Build history of the part. All positions in model axes, mm. Face numbers are marked on the shaded views. Round coordinates to 2 decimals unless told otherwise and drop trailing zeros. Order: outer loops, then holes, each group sorted by start corner. A loop starts at its lowest first (then second) coordinate and runs counter-clockwise, first axis right, second up. Notation, with made-up numbers: M -21.5,56 L -2.5,56 A24 ccw -2.5,88 Z; hole C -30.75,88 d3. An arc over 180 degrees is marked long. Use CSV: the item, a comma, the result in double quotes.
from build123d import *

# Parameters (mm, degrees)
PAD_DEPTH   = 40
SKETCH001_R = 5.5
HOLE_DEPTH  = 40.001


with BuildPart() as part:
    # Sketch → Pad (new body)
    with BuildSketch(Plane.XY):
        with BuildLine():
            Line((-17.5, 0), (-17.5, -17.5))
            Line((-17.5, -17.5), (17.5, -17.5))
            Line((17.5, -17.5), (17.5, 0))
            ThreePointArc((17.5, 0), (0, 17.5), (-17.5, 0))
        make_face()
    extrude(amount=PAD_DEPTH)

    # Sketch001 (on Face6 of Pad) → Hole (cut, through all)
    with BuildSketch(Plane.XY.offset(40)):
        with Locations((0, 2.5)):
            Circle(SKETCH001_R)
    extrude(amount=-HOLE_DEPTH, mode=Mode.SUBTRACT)


solid = part.part
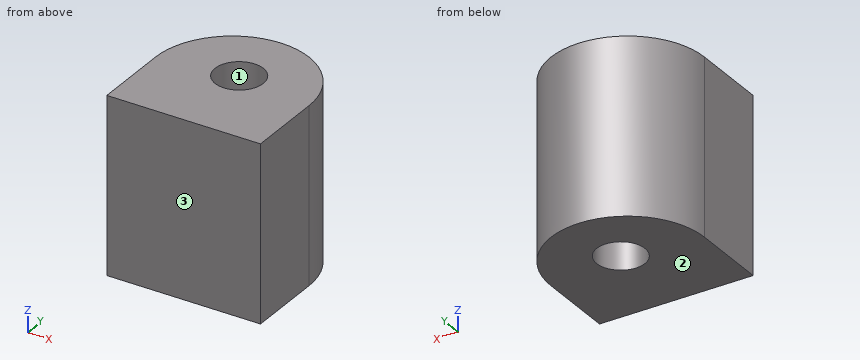
(1) Cut at B-B, the plane x = 0. Give the cut face in (y, z).
Answer block:
outline,"M -17.5,0 L -3,0 L -3,40 L -17.5,40 Z; M 8,0 L 17.5,0 L 17.5,40 L 8,40 Z"
(2) Wall check: line 1 (Y direction, x = 0, z = 9); line 2 (Y direction, x = -1, z = 30); line 3 (X direction, y = 2, z = 4.5). Give the ranges that are in metal, low to high. Write a range as from..to.
Answer block:
line 1,"y = -17.5..-3, 8..17.5"
line 2,"y = -17.5..-2.91, 7.91..17.47"
line 3,"x = -17.39..-5.48, 5.48..17.39"
(3) Two-plate mould, pull along Y, no slides. Class the marked faces 1, 2 and 3: released by +Y, released by -Y, zero draft, split by the parting line, or undercut.
Answer block:
face 1,"undercut"
face 2,"zero draft"
face 3,"released by -Y"
(4) Drop flat-ended pins along their axis: pin 1 (8 mm diameter, centred on y = 2, z = 7.5, fed in from +X); pin 2 (4 mm diameter, centred on x = -5, z = 8.5, fed in from +Y). Give the stop position or say it passes through.
Answer block:
pin 1,"stops at x = 17.5"
pin 2,"stops at y = 17.24"
(5) Cut at A-A, the plane z = 27. Give the cut face in (x, y), and give its area (3 significant figures).
Answer block:
outline,"M -17.5,-17.5 L 17.5,-17.5 L 17.5,0 A17.5 ccw -17.5,0 Z; hole C 0,2.5 d11"
area,"999 mm²"
(6) Cut at C-C, the plane y = 2.5. Give the cut face in (x, z), and give its area (3 significant figures).
Answer block:
outline,"M -17.32,0 L -5.5,0 L -5.5,40 L -17.32,40 Z; M 5.5,0 L 17.32,0 L 17.32,40 L 5.5,40 Z"
area,"946 mm²"
(7) Cut at D-D, the plane x = -10.5. Give the cut face in (y, z), and give its area (3 significant figures).
Answer block:
outline,"M -17.5,0 L 14,0 L 14,40 L -17.5,40 Z"
area,"1,260 mm²"
